```python
from build123d import *

# Parameters (mm, degrees)
SKETCH1_W           = 80
SKETCH1_H           = 80
BOSS_EXTRUDE1_DEPTH = 1.6
SKETCH5_R           = 3
CUT_EXTRUDE1_DEPTH  = 0.1
SKETCH6_R           = 1.6
CUT_EXTRUDE2_DEPTH  = 1.6


with BuildPart() as part:
    # Sketch1 → Boss-Extrude1 (new body)
    with BuildSketch(Plane(origin=(0, 0, 0), x_dir=(1, 0, 0), z_dir=(0, 1, 0))):
        Rectangle(SKETCH1_W, SKETCH1_H)
    extrude(amount=BOSS_EXTRUDE1_DEPTH)

    # Sketch5 → Cut-Extrude1 (cut)
    with BuildSketch(Plane(origin=(0, 1.6, 0), x_dir=(1, 0, 0), z_dir=(0, 1, 0))):
        with Locations((-36, 36)):
            Circle(SKETCH5_R)
        with Locations((36, 36)):
            Circle(SKETCH5_R)
        with Locations((36, -36)):
            Circle(SKETCH5_R)
        with Locations((-36, -36)):
            Circle(SKETCH5_R)
    extrude(amount=-CUT_EXTRUDE1_DEPTH, mode=Mode.SUBTRACT)

    # Sketch6 → Cut-Extrude2 (cut)
    with BuildSketch(Plane(origin=(0, 1.6, 0), x_dir=(1, 0, 0), z_dir=(0, 1, 0))):
        with Locations((-36, 36)):
            Circle(SKETCH6_R)
        with Locations((36, 36)):
            Circle(SKETCH6_R)
        with Locations((36, -36)):
            Circle(SKETCH6_R)
        with Locations((-36, -36)):
            Circle(SKETCH6_R)
    extrude(amount=-CUT_EXTRUDE2_DEPTH, mode=Mode.SUBTRACT)


solid = part.part
```
Can you work these out from the model? Positions are in its coordinate system, mm. A direction names the side the tool comes from. Coordinates: 2 decimals unless noted, no trailing zeros. Loops run counter-clockwise (first coordinate to the right, second up) from the corner with the lowest first, then second, coordinate; pieces in that order, holes last. Notation, with made-up numbers: (19, -25.75) - (28, -25.75) arc R21 cw to (28, -10.75) - close; hole circle Ø7 at (25, 71.5). An arc over 180 degrees is marked (long way). Answer as CSV lines item,"result". Start each with the question number.
1) Thinking about a two-plate mould opening in Z: for faces 3 (the cylindrical face through (34.73, 0.76, 36.97)), 4 (the cylindrical face through (-35.26, 0.76, 37.42)), 5 (the flat face through (-1, 0, -1)), which applies, pulls with the +Z half, pulls with the -Z half, needs draft (parallel to the pull), parting line crosses it, or undercut?
2) I need wall thicknesses on line 1 (X direction, y = 0.65, z = -36); line 2 (Z direction, x = 36, y = 1.55); line 3 (Z direction, x = 36.5, y = 0.1). Which ranges of each line are inside material? Lowest first, please. Write a range as from..to.
3) Suppose I cut it at A-A (x = 36). Please give me the cut outline in (y, z), plus the area to 3 significant figures.
4) Suppose I cut it at B-B (z = -36). Please give me the cut outline in (x, y).
5) Which directions (+Z, -Z, +X, -X, +Y, -Y) give clear straight access to the entire face, cutting with the end or side of a thin tool? Please do faces 1 (the flat face through (-1, 1.6, -1)), 2 (the flat face through (37.3, 1.5, 37.3)).
6) For pin 1 (5 mm diameter, centred on x = -36, z = 36, fed in from -Y); pin 2 (1.8 mm diameter, centred on x = -36.5, z = -37.5, fed in from +Y), each with a flat end and sliding along its axis, tell me the tip position at first contact or that it passes through.
Check result:
1,face 3,"undercut"
1,face 4,"undercut"
1,face 5,"needs draft"
2,line 1,"x = -40..-37.6, -34.4..34.4, 37.6..40"
2,line 2,"z = -40..-39, -33..33, 39..40"
2,line 3,"z = -40..-37.52, -34.48..34.48, 37.52..40"
3,outline,"(0, -40) - (1.6, -40) - (1.6, -39) - (1.5, -39) - (1.5, -37.6) - (0, -37.6) - close; (0, -34.4) - (1.5, -34.4) - (1.5, -33) - (1.6, -33) - (1.6, 33) - (1.5, 33) - (1.5, 34.4) - (0, 34.4) - close; (0, 37.6) - (1.5, 37.6) - (1.5, 39) - (1.6, 39) - (1.6, 40) - (0, 40) - close"
3,area,"117 mm²"
4,outline,"(-40, 0) - (-37.6, 0) - (-37.6, 1.5) - (-39, 1.5) - (-39, 1.6) - (-40, 1.6) - close; (-34.4, 0) - (34.4, 0) - (34.4, 1.5) - (33, 1.5) - (33, 1.6) - (-33, 1.6) - (-33, 1.5) - (-34.4, 1.5) - close; (37.6, 0) - (40, 0) - (40, 1.6) - (39, 1.6) - (39, 1.5) - (37.6, 1.5) - close"
5,face 1,"+Z, -Z, +X, -X, +Y"
5,face 2,"+Y"
6,pin 1,"stops at y = 0"
6,pin 2,"stops at y = 1.5"
